Design review of the part shown in the three views and the two pictorial views. Dimensions are in mm from the part's minimum x, y and z. Give positions to 0.01 mm unless a question says otherwise; leave off trailing zeros. Write each loop counter-clockwise with the first axis right and the second up, starting at its lowest first coordinate (ties: lowest second). Pieces come first, ordered by that corner, then holes.
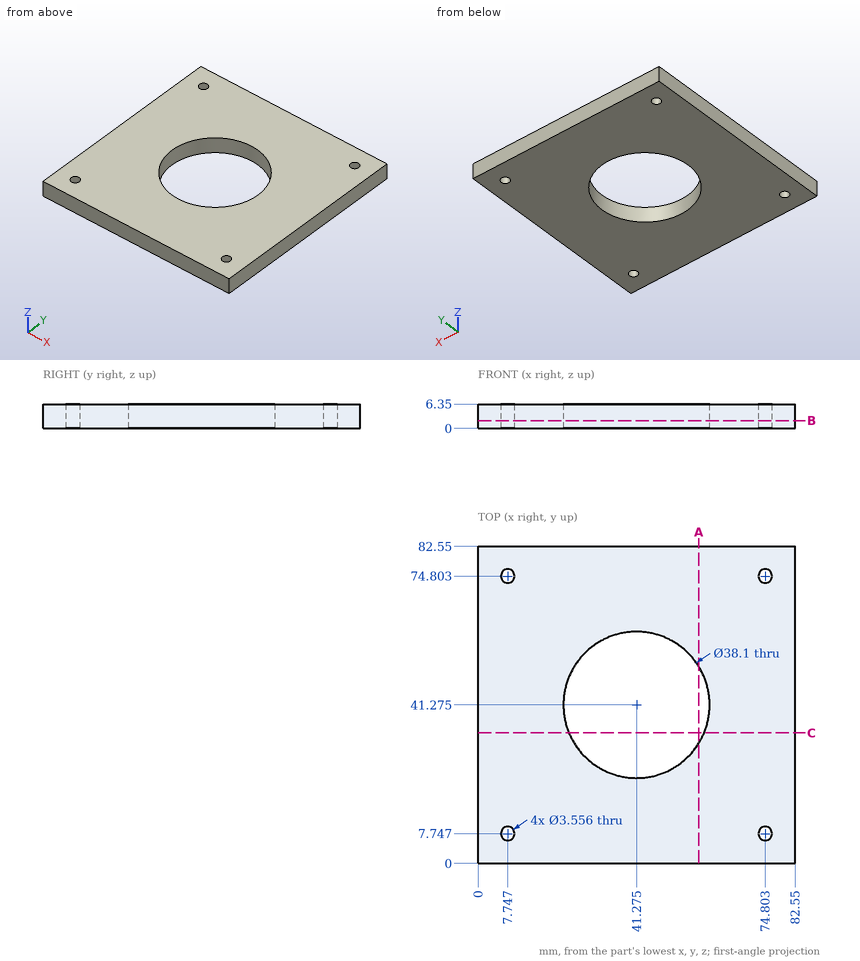
(1) Consider section C-C, the plane y = 34. Give the boundary of the cut face in (x, z).
Resolved:
outline: (0, 0) - (23.67, 0) - (23.67, 6.35) - (0, 6.35) - close; (58.88, 0) - (82.55, 0) - (82.55, 6.35) - (58.88, 6.35) - close
(2) To check wall thickness, follow L1, parallel to X at y = 40.5, z = 5.75; L2, parallel to X at y = 35, z = 2.75. State the ranges of each line that lie inside material, in increasing order.
Resolved:
L1: x = 0 to 22.24, 60.31 to 82.55
L2: x = 0 to 23.29, 59.26 to 82.55
(3) Consider section B-B, the plane z = 2. Give the boundary of the cut face in (x, y) (3 decimals).
Resolved:
outline: (0, 0) - (82.55, 0) - (82.55, 82.55) - (0, 82.55) - close; hole circle Ø3.556 at (7.747, 7.747); hole circle Ø3.556 at (7.747, 74.803); hole circle Ø38.1 at (41.275, 41.275); hole circle Ø3.556 at (74.803, 7.747); hole circle Ø3.556 at (74.803, 74.803)
(4) Consider section A-A, the plane x = 57.5. Give the boundary of the cut face in (y, z), then the cut area to 3 significant figures.
Resolved:
outline: (0, 0) - (31.29, 0) - (31.29, 6.35) - (0, 6.35) - close; (51.26, 0) - (82.55, 0) - (82.55, 6.35) - (51.26, 6.35) - close
area: 397 mm2
(5) Clearance check with a flat-ended pin moving along its axis: P1, Ø3, axis at x = 74.803, y = 7.747, coming from the +Z side. State where the tip first meets the part, or that it passes through.
Resolved:
P1: passes through
